Geometry: see drawing. Coordinates: mm, zero at the bounding-box minimum. A direction names the side the tool comes from. Coordinates: 2 decimals unless noted, no trailing zeros. Order: outer loops, then holes, each group sorted by start corner. A loop starts at its lowest first (then second) coordinate and runs counter-clockwise, first axis right, second up. Notation, with made-up numbers: (-1, -2) -> (12, -2) arc R30 cw to (12, 24) -> close; hole circle Ø6 at (-16.75, -2). An arc over 180 degrees is marked (long way). Use one line per item in the form item = value.
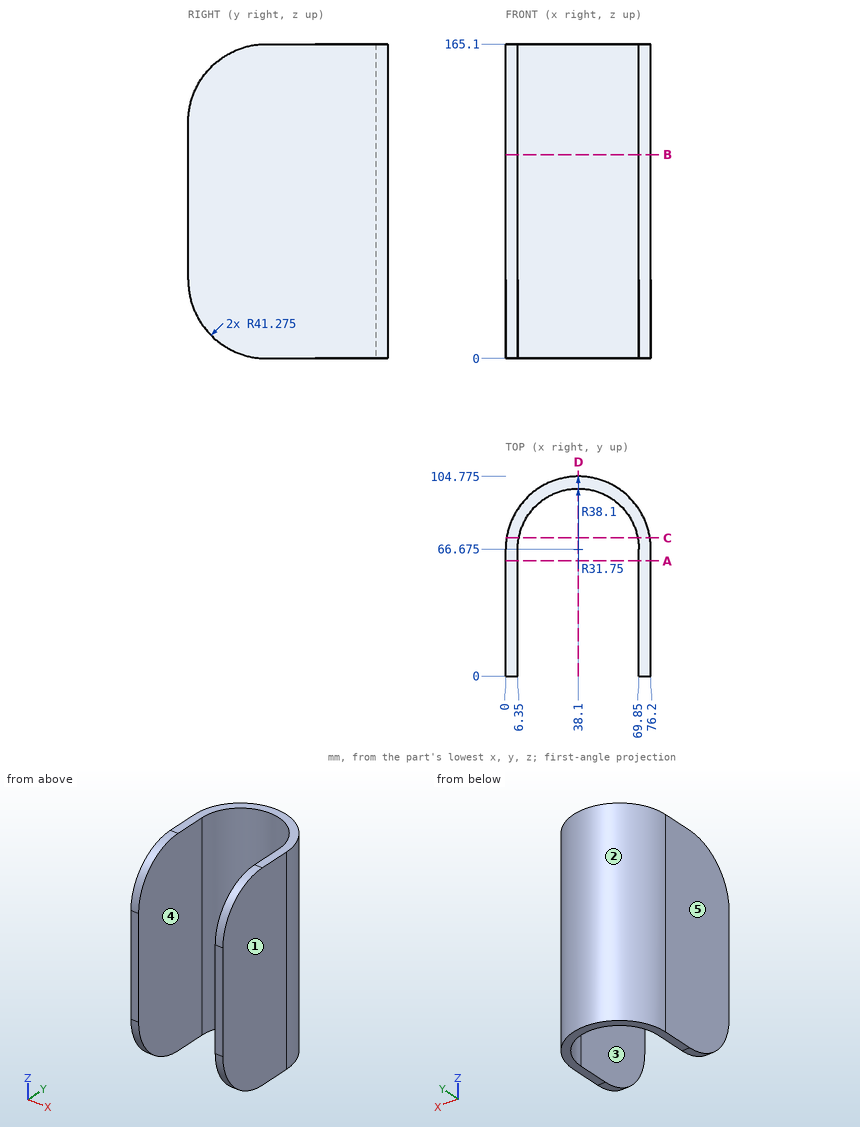
1) Section B-B, the plane z = 107. Output: boundary loops of the cut face in (x, y) (3 decimals), and give its area (3 significant figures).
Results found:
outline = (0, 0) -> (6.35, 0) -> (6.35, 66.675) arc R31.75 cw to (69.85, 66.675) -> (69.85, 0) -> (76.2, 0) -> (76.2, 66.675) arc R38.1 ccw to (0, 66.675) -> close
area = 1,540 mm2
2) Pull-direction query (X, two-part tool) for the marked faces 1, 2 and 3; classes: released by +X, released by -X, zero draft, split by the parting line, or undercut.
Results found:
face_1 = released by +X
face_2 = split by the parting line
face_3 = undercut
3) Section A-A, the plane y = 60.5. Output: boundary loops of the cut face in (x, z).
Results found:
outline = (0, 0) -> (6.35, 0) -> (6.35, 165.1) -> (0, 165.1) -> close; (69.85, 0) -> (76.2, 0) -> (76.2, 165.1) -> (69.85, 165.1) -> close
4) Contact query for flat-ended pins moving along their axis: P1, Ø10, axis at x = 46, z = 55.5, coming from the -Y side; P2, Ø6, axis at y = 78.5, z = 77.5, coming from the -X side; P3, Ø3, axis at x = 19, z = 47.5, coming from the -Y side. Output: stop coordinate, or through.
Results found:
P1 = 95.69
P2 = 1.04
P3 = 90.83
5) Access query for the marked faces 4 and 5. Directions: +Z, -Z, +X, -X, +Y, -Y. A direction counts if a zero-diameter tool reaches every point of the face in a straight line with its end or side. Return the directions, or none.
Results found:
face_4 = +Z, -Z, -Y
face_5 = +Z, -Z, -X, +Y, -Y
6) Material intervals for probe 1 along X at (y, z) = (18, 111); probe 2 along Y at (x, z) = (38.5, 72); probe 3 along X at (y, z) = (80, 150.5), sorted ascending. Write a range as from..to.
Results found:
probe_1 = 0..6.35, 69.85..76.2
probe_2 = 98.42..104.77
probe_3 = 2.41..9.28, 66.92..73.79
7) Section C-C, the plane y = 72.5. Output: boundary loops of the cut face in (x, z), and give its area (3 significant figures).
Results found:
outline = (0.45, 0) -> (6.89, 0) -> (6.89, 165.1) -> (0.45, 165.1) -> close; (69.31, 0) -> (75.75, 0) -> (75.75, 165.1) -> (69.31, 165.1) -> close
area = 2,130 mm2
8) Section D-D, the plane x = 38.1. Output: boundary loops of the cut face in (y, z) (3 decimals), and give its area (3 significant figures).
Results found:
outline = (98.425, 0) -> (104.775, 0) -> (104.775, 165.1) -> (98.425, 165.1) -> close
area = 1,050 mm2
